Source: CAD feature listing. Evaluate the final solid. Frame: model axes, mm. A direction names the side the tool comes from. Coordinates: 2 decimals unless noted, no trailing zeros. Loops run counter-clockwise (first coordinate to the right, second up) from the corner with the lowest first, then second, coordinate; pieces in that order, holes last. Notation, with made-up numbers: (64.5, 68.25) - (71.5, 68.25) arc R24 ccw to (71.5, 93.25) - close; hole circle Ø7 at (21.5, -28.75). An arc over 180 degrees is marked (long way). Use CSV: the item, a comma, the result in double quotes. Start each with the question number.
```python
from build123d import *

# Parameters (mm, degrees)
ESBO_O1_W                = 20
ESBO_O1_H                = 20
ESBO_O1_R                = 2
ESBO_O1_R_2              = 1.5
RESSALTO_EXTRUS_O1_DEPTH = 3
FILETE1_R                = 10
FILETE2_R                = 5


with BuildPart() as part:
    # Esboço1 → Ressalto-extrusão1 (new body)
    # profile 1 of 4: a face of its own
    with BuildSketch(Plane.XY):
        with Locations((10, 10)):
            Rectangle(ESBO_O1_W, ESBO_O1_H)
        with Locations((10, 10)):
            Circle(ESBO_O1_R, mode=Mode.SUBTRACT)
    # profile 2 of 4: a face of its own
    with BuildSketch(Plane.XY):
        with Locations((30, 10)):
            Rectangle(ESBO_O1_W, ESBO_O1_H)
        with Locations((30, 10)):
            Circle(ESBO_O1_R, mode=Mode.SUBTRACT)
    # profile 3 of 4: a face of its own
    with BuildSketch(Plane.XY):
        with Locations((30, 30)):
            Rectangle(ESBO_O1_W, ESBO_O1_H)
        with Locations((30, 30)):
            Circle(ESBO_O1_R, mode=Mode.SUBTRACT)
    # profile 4 of 4: a face of its own
    with BuildSketch(Plane.XY):
        with Locations((50, 30)):
            Rectangle(ESBO_O1_W, ESBO_O1_H)
        with Locations((50, 30)):
            Circle(ESBO_O1_R_2, mode=Mode.SUBTRACT)
    extrude(amount=RESSALTO_EXTRUS_O1_DEPTH)

    # Filete1
    filete1_edges = [part.edges().sort_by_distance(p)[0] for p in [
        (60, 20, 1.5),
        (60, 40, 1.5),
    ]]
    fillet(filete1_edges, radius=FILETE1_R - 0.0001)  # a hair under: the kernel refuses the full size

    # Filete2
    filete2_edges = [part.edges().sort_by_distance(p)[0] for p in [
        (20, 20, 1.5),
        (40, 20, 1.5),
    ]]
    fillet(filete2_edges, radius=FILETE2_R)


solid = part.part
```
(1) Section A-A on x = 30. Output: boundary loops of the cut face in (y, z), plus the area to 3 significant figures.
(2) Section D-D on x = 10. Output: boundary loops of the cut face in (y, z).
(3) Reachability of faces 1 (the cylindrical face through (30.923, 28.226, 1.479)), 2 (the flat face through (47, 20, 1)) from +Z, -Z, +X, -X, +Y, -Y: full face, straight path, thin tool, end or side. Return the list, or none.
(4) Draft query along X for faces 3 (the flat face through (20, 32, 1)), 4 (the cylindrical face through (31.908, 10.601, 1.479)), 5 (the flat face through (7, 20, 1)). Return one class per face: released by +X, released by -X, zero draft, split by the parting line, or undercut.
(5) Section B-B on z = 0.8. State how many separate pieces and enclosed holes the cut face has, plus the area to 3 significant figures.
(6) Ray query, line 1 (Y direction, x = 30, z = 2.25); line 2 (Y direction, x = 10, z = 2.65); line 3 (Y direction, x = 50, z = 2.15). Return the intervals inside material, ascending. Write a range as [from, to].
(7) Pin query (flat end, axial travel): pin 1 Ø2.5 at (x, y) = (30, 30) entering from -Z; pin 2 Ø3.5 at (x, y) = (50, 30) entering from +Z; pin 3 Ø0.9 at (y, z) = (31.5, 2) entering from -X; pin 4 Ø1.5 at (x, z) = (46.5, 1) entering from -Y. Return the tip coordinate at first contact, or that it passes through.
Solution:
1,outline,"(0, 0) - (8, 0) - (8, 3) - (0, 3) - close; (12, 0) - (28, 0) - (28, 3) - (12, 3) - close; (32, 0) - (40, 0) - (40, 3) - (32, 3) - close"
1,area,"96.0 mm²"
2,outline,"(0, 0) - (8, 0) - (8, 3) - (0, 3) - close; (12, 0) - (20, 0) - (20, 3) - (12, 3) - close"
3,face 1,"+Z, -Z"
3,face 2,"+Z, -Z, +X, -Y"
4,face 3,"released by -X"
4,face 4,"undercut"
4,face 5,"zero draft"
5,separate pieces,"1"
5,enclosed holes,"4"
5,area,"1,520 mm²"
6,line 1,"y = [0, 8], [12, 28], [32, 40]"
6,line 2,"y = [0, 8], [12, 20]"
6,line 3,"y = [20, 28.5], [31.5, 40]"
7,pin 1,"passes through"
7,pin 2,"stops at z = 3"
7,pin 3,"stops at x = 20"
7,pin 4,"stops at y = 20"
